Can you work these out from the model? Positions are in its coordinate system, mm. A direction names the side the tool comes from. Give positions to 0.01 mm unless a question says otherwise; leave off trailing zeros. Order: outer loops, then holes, each group sorted by start corner. A loop starts at its lowest first (then second) coordinate and runs counter-clockwise, first axis right, second up.
Autodesk Inventor part; units mm, degrees
ref_plane "YZ Plane" through (0, 0, 0) normal (1, 0, 0) x (0, 1, 0)
ref_plane "XZ Plane" through (0, 0, 0) normal (0, 1, 0) x (-1, 0, 0)
ref_plane "XY Plane" through (0, 0, 0) normal (0, 0, 1) x (1, 0, 0)
sketch "Sketch1" plane through (0, 0, 0) normal (0, 0, 1) x (1, 0, 0)
  line L0 (0, 17.4) -> (0, -20.4) construction
  line L1 (-20.2396, 0) -> (20.2396, 0) construction
  circle A0 centre (0, 0) radius 5.5
  circle A1 centre (0, 8) radius 2
  arc A2 (-14.4568, -4) -> (14.4568, -4) centre (0, 0) ccw
  line L2 (-14.4568, -4) -> (-5.5, 0)
  line L3 (5.5, 0) -> (14.4568, -4)
  line L4 (-3.9291, 8.7499) -> (-5.3921, 1.0839)
  line L5 (3.9291, 8.7499) -> (5.3921, 1.0839)
  arc A3 (3.9291, 8.7499) -> (-3.9291, 8.7499) centre (0, 8) ccw
  circle A4 centre (0, 0) radius 4
  arc A5 (5.3921, 1.0839) -> (-5.3921, 1.0839) centre (0, 0) ccw
  dimension "d0" = 11
  dimension "d1" = 4
  dimension "d3" = 8
  dimension "d4" = 15
  dimension "d5" = 4
  dimension "d7" = 21.61
  dimension "d8" = 4
  dimension "d21" = 8
extrude "Extrusion1" add sketch "Sketch1" along normal mid plane 6 contours L3 A2 L2 A0 | A0 L4 A3 L5
extrude "Extrusion2" add sketch "Sketch1" along normal blind 3.5 contours A0
extrude "Extrusion3" add sketch "Sketch1" against normal up to surface (3 mm away) contours A0
sketch "Sketch2" plane through (0, 0, 3.5) normal (0, 0, 1) x (1, 0, 0)
  circle A0 centre (0, 0) radius 4 construction
  circle A1 centre (0, 0) radius 5.5 construction
  circle A2 centre (0, 4) radius 0.5
  dimension "d16" = 1
extrude "Extrusion4" cut sketch "Sketch2" against normal through all
extrude "Extrusion5" add sketch "Sketch1" against normal blind 10 contours A1
extrude "Extrusion6" add sketch "Sketch1" along normal up to surface (3 mm away) contours A1
sketch "Sketch3" plane through (0, 8, -10) normal (0, 0, -1) x (-1, 0, 0)
  circle A0 centre (0, 0) radius 2 construction
  circle A1 centre (0, 0) radius 2
  circle A2 centre (0, 0) radius 2
  circle A3 centre (0, 0) radius 2.5
  arc A4 (5.3921, -6.9161) -> (-5.3921, -6.9161) centre (0, -8) ccw
extrude "Extrusion7" add sketch "Sketch3" against normal blind 0.5
properties part number "Crank" material "Iron, Cast"
1) Suppose I cut it at D-D (z = -4). Please give me the cut outline in (x, y), and give its area (3 significant figures).
2) Which directions (+Z, -Z, +X, -X, +Y, -Y) give clear straight access to the entire face, cutting with the end or side of a thin tool? Please do faces 4 (the face through (0, 8, 3)), 5 (the face through (0, 4.5, 0.3)), 6 (the face through (0.54, 5.56, -9.75)), 7 (the face through (5.47, 0.56, 1.71)).
3) If I drill on line 1 (Y direction, x = 0, z = -0.25); line 2 (Z direction, x = -9.5, y = -11.5); line 3 (Y direction, x = -0.75, z = 1.25), over which ranges is the centre line in solid material (lowest first)?
4) I'm going to push flat-ended pins straight in: pin 1 Ø4 at (x, z) = (2.5, -8) entering from +Y; pin 2 Ø3 at (x, y) = (-2, 7.5) entering from +Z; pin 3 Ø12 at (x, y) = (8, -2.5) entering from -Z; pin 4 Ø7 at (x, y) = (0, 0) entering from -Z. Where does each tip first touch, or does it pass through?
5) Suppose I cut it at A-A (x = 0). Please give me the cut outline in (y, z), and give its area (3 significant figures).
6) Suppose I cut it at C-C (z = -2.5). Please give me the cut outline in (x, y).
7) We'd pull the mould along Z, two halves only. Please class faces 1 (the face through (0, -7, 3)), 2 (the face through (9.916, -1.972, -0.042)), 3 (the face through (1, 10, -9.5)): +Z half, -Z half, draft (parallel to the pull), parting line (faces both ways), or undercut.
Results:
1. outline: circle Ø4 at (0, 8)
1. area: 12.6 mm2
2. face 4: +Z, +Y
2. face 5: +Z, -Z
2. face 6: -Z
2. face 7: +Z
3. line 1: y = -15 to -4, 4.5 to 12
3. line 2: z = -3 to 3
3. line 3: y = -14.98 to -3.93, 3.93 to 11.93
4. pin 1: stops at y = 10.21
4. pin 2: stops at z = 3
4. pin 3: stops at z = -3
4. pin 4: passes through
5. outline: (-15, -3) - (-4, -3) - (-4, 3.5) - (-5.5, 3.5) - (-5.5, 3) - (-15, 3) - close; (4.5, -3) - (6, -3) - (6, -9.5) - (5.5, -9.5) - (5.5, -10) - (10.5, -10) - (10.5, -9.5) - (10, -9.5) - (10, -3) - (12, -3) - (12, 3) - (5.5, 3) - (5.5, 3.5) - (4.5, 3.5) - close
5. area: 141 mm2
6. outline: (-14.46, -4) arc R15 ccw to (14.46, -4) - (5.5, 0) arc R5.5 ccw to (5.39, 1.08) - (3.93, 8.75) arc R4 ccw to (-3.93, 8.75) - (-5.39, 1.08) arc R5.5 ccw to (-5.5, 0) - close; hole (-0.5, 3.97) arc R4 ccw (long way) to (0.5, 3.97) arc R0.5 ccw (long way) to start
7. face 1: +Z half
7. face 2: draft
7. face 3: undercut
